Answer from the drawing. Dimensions are ordinates in mm from the lowest x, y and z of the part. Coordinates: 2 decimals unless noted, no trailing zeros. Write each loop counter-clockwise with the first axis right and the second up, starting at its lowest first coordinate (ties: lowest second). Pieces come first, ordered by that corner, then holes. Notation, with made-up numbers: (85, -9.5) - (142, -9.5) arc R19 ccw to (142, 15.5) - close; hole circle Ø10 at (-30, 84.5). An arc over 180 degrees is marked (long way). Answer as a JSON object with one key per item and string values. Group by question number.
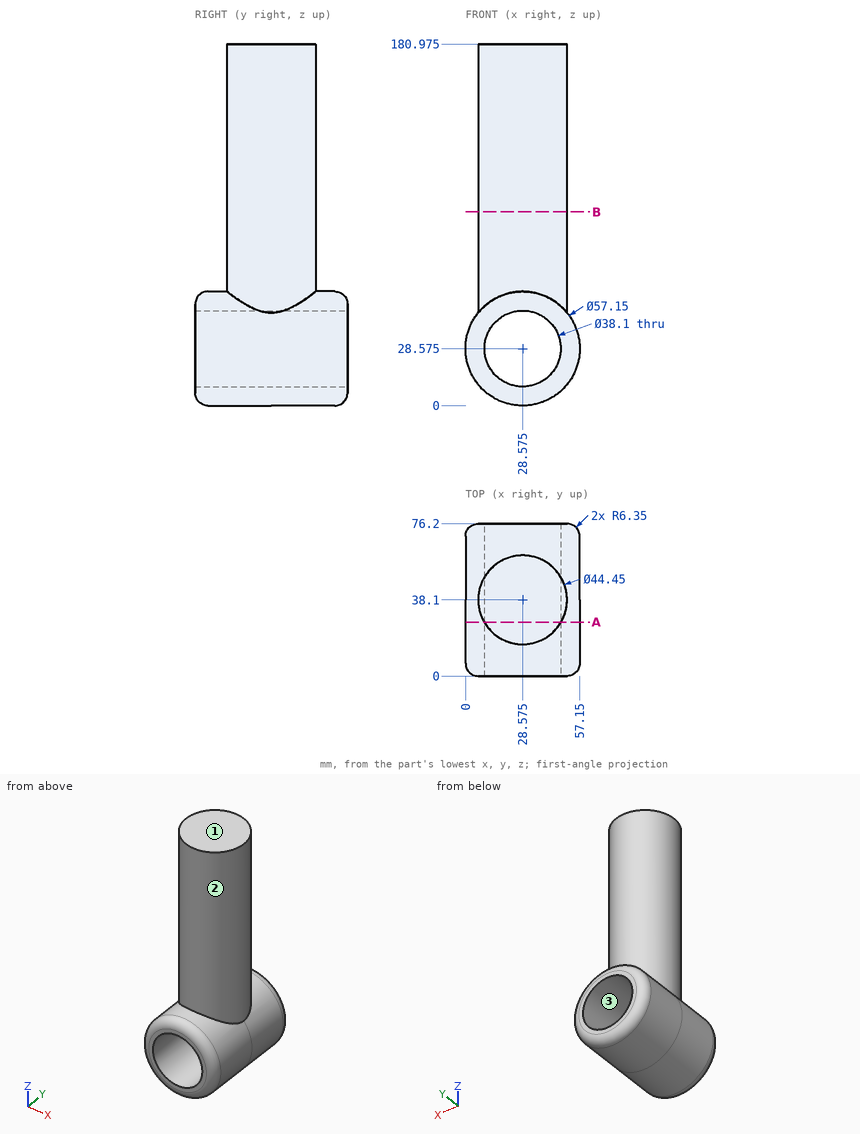
Q1. Consider L1, parallel to X at y = 56.5, z = 40.5; L2, parallel to Z at x = 18, y = 40 (3 decimals); L3, parallel to Y at x = 51, z = 29. Determine where each line is inside the solid, lowest interval first. Write a range as from..to.
Q2. For a pull along Z with two mould halves and no side action, classify the marked faces 1, 2 and 3 as +Z half, -Z half, draft (parallel to the pull), parting line (faces both ways), or undercut.
Q3. Section B-B on z = 97 is taken. Determine the outline of the cut face in (x, y) (3 decimals).
Q4. Section A-A on y = 27 is taken. Determine the outline of the cut face in (x, z) (3 decimals).
Q5. Flat-ended cylindrical pins translate along their axes: pin 1 Ø8 at (x, z) = (9, 150) entering from +Y; pin 2 Ø5 at (x, z) = (47, 156.5) entering from +Y; pin 3 Ø2 at (y, z) = (28, 43) entering from +X. Find the tip coordinate at first contact, or state that the pin passes through.
Numbers:
{
 "1": {"L1": "x = 2.61..13.72, 43.43..54.54", "L2": "z = 2.029..12.73, 44.42..180.975", "L3": "y = 0..76.2"},
 "2": {"face 1": "+Z half", "face 2": "draft", "face 3": "undercut"},
 "3": {"outline": "circle Ø44.45 at (28.575, 38.1)"},
 "4": {"outline": "(9.32, 49.689) arc R28.575 ccw (long way) to (47.83, 49.689) - (47.83, 180.975) - (9.32, 180.975) - close; hole circle Ø38.1 at (28.575, 28.575)"},
 "5": {"pin 1": "stops at y = 53.95", "pin 2": "stops at y = 53.6", "pin 3": "stops at x = 53.8"}
}
